Study the drawing (mm; zero at the part's minimum x, y, z) and answer. A direction names the side the tool comes from. Round coordinates to 2 decimals unless told otherwise and drop trailing zeros. Write each loop counter-clockwise with the first axis right and the second up, starting at its lowest first coordinate (ties: lowest second). Pieces come first, ordered by that corner, then holes.
(1) A cutting plane is placed at C-C, the plane y = 42.5. Give the vertices of the cut face in (x, z).
(2) A cutting plane is placed at A-A, the plane z = 39. Give the vertices of the cut face in (x, y) (1 decimal).
(3) A cutting plane is placed at D-D, the plane x = 22.5. Give the vertices of the cut face in (y, z), and give its area (3 significant figures).
(4) Each of these flat-tipped pins is pushed along its axis until it touches: pin 1 Ø2.5 at (x, z) = (56.5, 45.5) entering from +Y; pin 2 Ø3 at (y, z) = (66, 70) entering from +X; pin 3 Ø24 at (y, z) = (68.5, 47) entering from -X; pin 4 Ø5.5 at (x, y) = (55.5, 64.5) entering from -Z. Where does it stop, or does it pass through?
(5) A cutting plane is placed at B-B, the plane z = 74. Give the vertices of the cut face in (x, y) (1 decimal).
(6) For the marked faces 1 and 2, determine the directions among +Z, -Z, +X, -X, +Y, -Y from which every point of the face is accessible in a straight line to the end or side of a thin tool.
(7) Find the intervals of material crossed by probe 1 along Z at (x, y) = (46, 98); probe 2 along X at (y, z) = (91, 79.5); probe 3 along X at (y, z) = (16.5, 83), in increasing order.
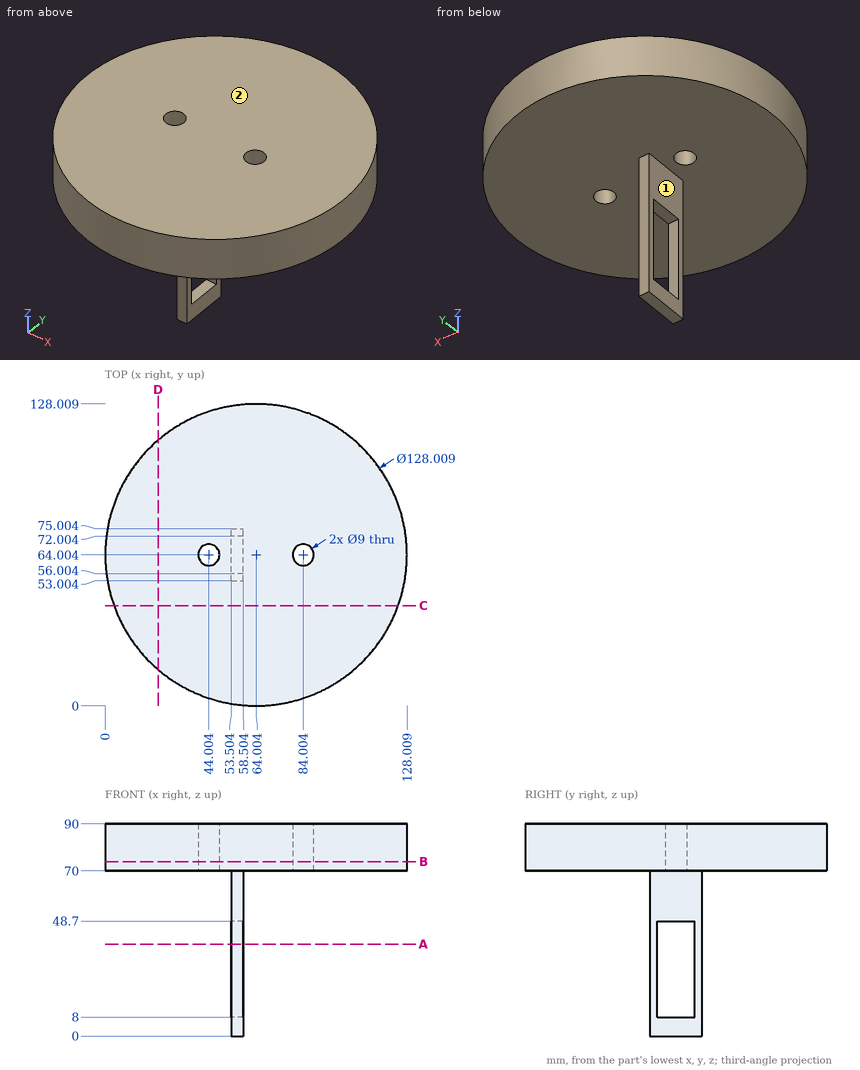
Solutions:
1. outline: (3.72, 70) - (124.29, 70) - (124.29, 90) - (3.72, 90) - close
2. outline: (53.5, 53) - (58.5, 53) - (58.5, 56) - (53.5, 56) - close; (53.5, 72) - (58.5, 72) - (58.5, 75) - (53.5, 75) - close
3. outline: (15.28, 70) - (112.73, 70) - (112.73, 90) - (15.28, 90) - close
3. area: 1,950 mm2
4. pin 1: stops at y = 75
4. pin 2: stops at x = 128.01
4. pin 3: stops at x = 53.5
4. pin 4: stops at z = 0
5. outline: circle Ø128 at (64, 64); hole circle Ø9 at (44, 64); hole circle Ø9 at (84, 64)
6. face 1: -Z, -X, +Y, -Y
6. face 2: +Z, +X, -X, +Y, -Y
7. probe 1: z = 70 to 90
7. probe 2: x = 5.97 to 122.04
7. probe 3: x = 21.11 to 106.9
